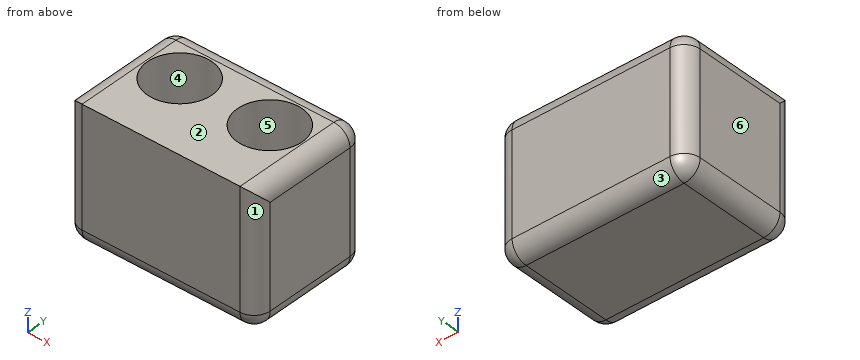
```python
from build123d import *

# Parameters (mm, degrees)
ESBO_O1_W                = 17.7
ESBO_O1_H                = 11.5
RESSALTO_EXTRUS_O1_DEPTH = 12.5
ESBO_O2_R                = 3
CORTE_EXTRUS_O1_DEPTH    = 10
FILETE1_R                = 1.5


with BuildPart() as part:
    # Esboço1 → Ressalto-extrusão1 (new body)
    with BuildSketch(Plane.XY):
        Rectangle(ESBO_O1_W, ESBO_O1_H)
    extrude(amount=RESSALTO_EXTRUS_O1_DEPTH)

    # Esboço2 → Corte-extrusão1 (cut)
    with BuildSketch(Plane.XY.offset(12.5)):
        with Locations((4.195, 1.04)):
            Circle(ESBO_O2_R)
        with Locations((-4.195, 1.04)):
            Circle(ESBO_O2_R)
    extrude(amount=-CORTE_EXTRUS_O1_DEPTH, mode=Mode.SUBTRACT)

    # Filete1
    filete1_edges = [part.edges().sort_by_distance(p)[0] for p in [
        (-8.85, 0, 12.5),
        (8.85, 0, 12.5),
        (0, -5.75, 0),
        (-8.85, 0, 0),
        (0, 5.75, 0),
        (8.85, 0, 0),
        (8.85, -5.75, 6.25),
        (-8.85, -5.75, 6.25),
        (-8.85, 5.75, 6.25),
        (8.85, 5.75, 6.25),
        (0, 5.75, 12.5),
    ]]
    fillet(filete1_edges, radius=FILETE1_R)


solid = part.part
```
Geometry: final body of the model. Coordinates: model frame, mm. Face numbers are marked on the shaded views. A direction names the side the tool comes from. Round coordinates to 2 decimals unless told otherwise and drop trailing zeros. Write each loop counter-clockwise with the first axis right and the second up, starting at its lowest first coordinate (ties: lowest second). Pieces come first, ordered by that corner, then holes. Notation, with made-up numbers: M 24,6.5 L 52,6.5 A13 ccw 52,25.5 Z; hole C 54.25,-7 d4. An arc over 180 degrees is marked long. Answer in a Markdown table with one row per item. Add a question column.
(1) Ray query, L1, parallel to X at y = -0.25, z = 6.5; L2, parallel to X at y = -1.25, z = 8.75; L3, parallel to Y at x = -4.5, z = 11. Return the intervals inside material, ascending.
(2) Reachability of the marked faces 5 and 6 from +Z, -Z, +X, -X, +Y, -Y: full face, straight path, thin tool, end or side. Return the list, or none.
(3) Draft query along Y for the marked faces 1, 2, 3 and 4. Return one class per face: pulls with the +Y half, pulls with the -Y half, needs draft (parallel to the pull), parting line crosses it, or undercut.
(4) Cut plane A-A, the plane z = 4.75. Return the cut outline in (x, y) (3 decimals).
(5) Cut plane D-D, the plane z = 1.25. Return the cut outline in (x, y).
(6) Cut plane B-B, the plane y = 1.04. Return the cut outline in (x, z) (3 decimals), then the cut area to 3 significant figures.
(7) Contact query for a flat-ended pin moving along its axis: pin 1 (1.8 mm diameter, centred on x = 5, y = 1, fed in from +Z). Output: stop coordinate, or through.
(8) Cut plane C-C, the plane x = 5.25. Return the cut outline in (y, z), then the cut area to 3 significant figures.
Established:
| question | item | result |
|---|---|---|
| 1 | L1 | -8.85 to -6.9, -1.49 to 1.49, 6.9 to 8.85 |
| 1 | L2 | -8.85 to -6.13, -2.26 to 2.26, 6.13 to 8.85 |
| 1 | L3 | -5.75 to -1.94, 4.02 to 5.75 |
| 2 | face 5 | +Z |
| 2 | face 6 | +Z, -Z, -X, +Y, -Y |
| 3 | face 1 | pulls with the -Y half |
| 3 | face 2 | needs draft |
| 3 | face 3 | pulls with the +Y half |
| 3 | face 4 | undercut |
| 4 | outline | M -8.85,-4.25 A1.5 ccw -7.35,-5.75 L 7.35,-5.75 A1.5 ccw 8.85,-4.25 L 8.85,4.25 A1.5 ccw 7.35,5.75 L -7.35,5.75 A1.5 ccw -8.85,4.25 Z; hole C -4.195,1.04 d6; hole C 4.195,1.04 d6 |
| 5 | outline | M -8.83,-4.25 A1.48 ccw -7.35,-5.73 L 7.35,-5.73 A1.48 ccw 8.83,-4.25 L 8.83,4.25 A1.48 ccw 7.35,5.73 L -7.35,5.73 A1.48 ccw -8.83,4.25 Z |
| 6 | outline | M -8.85,1.5 A1.5 ccw -7.35,0 L 7.35,0 A1.5 ccw 8.85,1.5 L 8.85,11 A1.5 ccw 7.35,12.5 L 7.195,12.5 L 7.195,2.5 L 1.195,2.5 L 1.195,12.5 L -1.195,12.5 L -1.195,2.5 L -7.195,2.5 L -7.195,12.5 L -7.35,12.5 A1.5 ccw -8.85,11 Z |
| 6 | area | 99.3 mm² |
| 7 | pin 1 | z = 2.5 |
| 8 | outline | M -5.75,1.5 A1.5 ccw -4.25,0 L 4.25,0 A1.5 ccw 5.75,1.5 L 5.75,11 A1.5 ccw 4.25,12.5 L 3.85,12.5 L 3.85,2.5 L -1.77,2.5 L -1.77,12.5 L -5.75,12.5 Z |
| 8 | area | 86.1 mm² |
